Input: part model. Units: mm. Frame: model coordinates. A direction names the side the tool comes from. Round coordinates to 2 decimals unless told otherwise and drop trailing zeros. Write each loop counter-clockwise with the first axis right and the second up, starting at its lowest first coordinate (ties: lowest second). Pieces come first, ordered by that corner, then holes. Notation, with made-up numbers: (54, -37.5) - (113, -37.5) arc R25 ccw to (113, -23.5) - close; hole circle Ø5 at (16, 71). An arc over 180 degrees is marked (long way). Use one line per item in the form item = value.
```python
from build123d import *

# Parameters (mm, degrees)
BOSS_EXTRUDE1_DEPTH = 72
BOSS_EXTRUDE3_DEPTH = 5
CUT_EXTRUDE4_DEPTH  = 5
BOSS_EXTRUDE4_DEPTH = 5
BOSS_EXTRUDE5_START = 7
BOSS_EXTRUDE5_DEPTH = 55
CUT_EXTRUDE8_DEPTH  = 5
SKETCH19_W          = 15
SKETCH19_H          = 12.25
BOSS_EXTRUDE8_DEPTH = 7
CUT_EXTRUDE9_REACH  = 78.51
SKETCH20_R          = 1.5
SKETCH21_W          = 23.7
SKETCH21_H          = 22.72285099
CUT_EXTRUDE10_DEPTH = 7
SKETCH24_W          = 13.67
SKETCH24_H          = 10.75
CUT_EXTRUDE13_DEPTH = 65


with BuildPart() as part:
    # Sketch1 → Boss-Extrude1 (new body)
    with BuildSketch(Plane.XY):
        Polygon((-14.835, 0), (-6.835, 0), (-6.835, 3), (6.835, 3), (6.835, 0), (14.835, 0), (14.835, 4.5), (8.35, 4.5), (-8.35, 4.5), (-14.835, 4.5), align=None)
    extrude(amount=-BOSS_EXTRUDE1_DEPTH)

    # Sketch8 → Boss-Extrude3 (add)
    with BuildSketch(Plane(origin=(0, 0, -72), x_dir=(-1, 0, 0), z_dir=(0, 0, -1))):
        Polygon((-14.835, 25.70785099), (-14.835, 0), (-10.35, 0), (-10.35, 21.22285099), (10.35, 21.22285099), (10.35, 0), (14.835, 0), (14.835, 25.70785099), align=None)
    extrude(amount=-BOSS_EXTRUDE3_DEPTH)

    # Sketch9 → Cut-Extrude4 (cut)
    with BuildSketch(Plane(origin=(0, 0, -72), x_dir=(-1, 0, 0), z_dir=(0, 0, -1))):
        with BuildLine():
            Line((-15.009070225, 25.881921215), (-15.009070225, 22.527488279))
            ThreePointArc((-15.009070225, 22.527488279), (-13.436955933, 24.309806923), (-11.654637289, 25.881921215))
            Line((-11.654637289, 25.881921215), (-15.009070225, 25.881921215))
        make_face()
        with BuildLine():
            Line((15.009070225, 25.881921215), (15.009070225, 22.527488279))
            ThreePointArc((15.009070225, 22.527488279), (13.436955933, 24.309806923), (11.654637289, 25.881921215))
            Line((11.654637289, 25.881921215), (15.009070225, 25.881921215))
        make_face()
    extrude(amount=-CUT_EXTRUDE4_DEPTH, mode=Mode.SUBTRACT)

    # Sketch11 → Boss-Extrude4 (add)
    with BuildSketch(Plane.XY.offset(-67)):
        with BuildLine():
            Line((14.835, 4.5), (14.835, 22.748275799))
            ThreePointArc((14.835, 22.748275799), (13.436955933, 24.309806923), (11.875424809, 25.70785099))
            Line((11.875424809, 25.70785099), (-11.875424809, 25.70785099))
            ThreePointArc((-11.875424809, 25.70785099), (-13.436955933, 24.309806923), (-14.835, 22.748275799))
            Line((-14.835, 22.748275799), (-14.835, 4.5))
            Line((-14.835, 4.5), (14.835, 4.5))
        make_face()
    extrude(amount=BOSS_EXTRUDE4_DEPTH)

    # Sketch12 → Boss-Extrude5 (add)
    with BuildSketch(Plane.XY.offset(-62).offset(BOSS_EXTRUDE5_START)):
        with BuildLine():
            Line((-14.835, 4.5), (14.832662348, 4.5))
            Line((14.832662348, 4.5), (14.832662348, 9.600169894))
            ThreePointArc((14.832662348, 9.600169894), (12.620742321, 14.666687642), (7.5, 16.75))
            Line((7.5, 16.75), (-7.5, 16.75))
            ThreePointArc((-7.5, 16.75), (-12.68662824, 14.60162824), (-14.835, 9.415))
            Line((-14.835, 9.415), (-14.835, 4.5))
        make_face()
    extrude(amount=BOSS_EXTRUDE5_DEPTH)

    # Sketch18 → Cut-Extrude8 (cut)
    with BuildSketch(Plane(origin=(0, 0, -72), x_dir=(-1, 0, 0), z_dir=(0, 0, -1))):
        Polygon((-10.35, 4.5), (-10.35, 0), (-6.835, 0), (-6.835, 3), (6.835, 3), (6.835, 0), (10.35, 0), (10.35, 4.5), align=None)
    extrude(amount=-CUT_EXTRUDE8_DEPTH, mode=Mode.SUBTRACT)

    # Sketch19 → Boss-Extrude8 (add)
    with BuildSketch(Plane(origin=(0, 0, -55), x_dir=(-1, 0, 0), z_dir=(0, 0, -1))):
        with Locations((0, 10.625)):
            Rectangle(SKETCH19_W, SKETCH19_H)
    extrude(amount=BOSS_EXTRUDE8_DEPTH)

    # Sketch20 → Cut-Extrude9 (cut, up to next)
    with BuildSketch(Plane(origin=(0, 4.5, 0), x_dir=(1, 0, 0), z_dir=(0, 1, 0)), mode=Mode.PRIVATE) as cut_extrude9_sk1:
        with Locations(Location((-10.5425, 58.5, 0), (0, 0, 180))):
            Circle(SKETCH20_R)
    cut_extrude9_tool1 = extrude(cut_extrude9_sk1.sketch, amount=-CUT_EXTRUDE9_REACH, mode=Mode.PRIVATE) & part.part
    # Sketch20 → Cut-Extrude9 (cut, up to next)
    with BuildSketch(Plane(origin=(0, 4.5, 0), x_dir=(1, 0, 0), z_dir=(0, 1, 0)), mode=Mode.PRIVATE) as cut_extrude9_sk2:
        with Locations(Location((10.5425, 58.5, 0), (0, 0, 270))):
            Circle(SKETCH20_R)
    cut_extrude9_tool2 = extrude(cut_extrude9_sk2.sketch, amount=-CUT_EXTRUDE9_REACH, mode=Mode.PRIVATE) & part.part
    add(cut_extrude9_tool1.solids().sort_by_distance((-10.5425, 4.5, -58.5))[0], mode=Mode.SUBTRACT)
    add(cut_extrude9_tool2.solids().sort_by_distance((10.5425, 4.5, -58.5))[0], mode=Mode.SUBTRACT)

    # Sketch21 → Cut-Extrude10 (cut)
    with BuildSketch(Plane(origin=(0, 0, -72), x_dir=(-1, 0, 0), z_dir=(0, 0, -1))):
        with Locations((0, 11.361425495)):
            Rectangle(SKETCH21_W, SKETCH21_H)
    extrude(amount=-CUT_EXTRUDE10_DEPTH, mode=Mode.SUBTRACT)

    # Sketch24 → Cut-Extrude13 (cut)
    with BuildSketch(Plane.XY):
        with Locations((0, 8.375)):
            Rectangle(SKETCH24_W, SKETCH24_H)
    extrude(amount=-CUT_EXTRUDE13_DEPTH, mode=Mode.SUBTRACT)


solid = part.part
```
(1) Cut plane C-C on x = -10.25. Output: boundary loops of the cut face in (y, z), then the cut area to 3 significant figures.
Derived:
outline = (0, -65) - (22.72, -65) - (22.72, -72) - (25.71, -72) - (25.71, -62) - (4.5, -62) - (4.5, -59.97) - (0, -59.97) - close; (0, -57.03) - (4.5, -57.03) - (4.5, -55) - (16.21, -55) - (16.21, 0) - (0, 0) - close
area = 1,010 mm^2
(2) First-contact query: pin 1 Ø1.5 at (x, z) = (3, -59.5) entering from -Y; pin 2 Ø3.5 at (x, y) = (10, 7.5) entering from -Z; pin 3 Ø1.5 at (x, z) = (6, -52) entering from +Y. Flat tips, straight axial feed; report the tip coordinate or a pass-through.
Derived:
pin_1 = 13.75
pin_2 = -65
pin_3 = 16.75
(3) Material intervals for L1, parallel to Z at x = -10.5, y = 16; L2, parallel to X at y = 1.5, z = -9 (3 decimals); L3, parallel to Z at x = -11.5, y = 21.5, sorted ascending.
Derived:
L1 = -65 to -62, -55 to 0
L2 = -14.835 to -6.835, 6.835 to 14.835
L3 = -65 to -62
(4) Cut plane A-A on z = -58.5. Count the separate pieces of the cut face and the enclosed holes in it, then the cut area to 3 significant figures.
Derived:
separate_pieces = 3
enclosed_holes = 0
area = 102 mm^2
(5) Access query for faces 4 (the face through (0, 16.75, -31)), 5 (the face through (0, 22.723, -69)), 6 (the face through (0, 13.75, -32)), 7 (the face through (-12.63, 14.66, -27.88)), 8 (the face through (12.3, 4.5, -58.4)). Directions: +Z, -Z, +X, -X, +Y, -Y. A direction counts if a zero-diameter tool reaches every point of the face in a straight line with its end or side. Return the directions, or none.
Derived:
face_4 = +Z, +X, -X, +Y
face_5 = -Z, -Y
face_6 = +Z, -Z, -Y
face_7 = +Z, -X, +Y
face_8 = +X, +Y
(6) Draft query along X for faces 1 (the face through (6.835, 7, -32)), 2 (the face through (0, 18, -62)), 3 (the face through (7.5, 11, -58)). Return one class per face: released by +X, released by -X, zero draft, split by the parting line, or undercut.
Derived:
face_1 = undercut
face_2 = zero draft
face_3 = released by +X
(7) Cut plane B-B on y = 5.5. Output: boundary loops of the cut face in (x, z) (3 decimals).
Derived:
outline = (-14.835, -72) - (-11.85, -72) - (-11.85, -65) - (-6.835, -65) - (-6.835, 0) - (-14.835, 0) - (-14.835, -55) - (-7.5, -55) - (-7.5, -62) - (-14.835, -62) - close; (6.835, -65) - (11.85, -65) - (11.85, -72) - (14.835, -72) - (14.835, -62) - (7.5, -62) - (7.5, -55) - (14.833, -55) - (14.833, 0) - (6.835, 0) - close
